Verification items for the finished model (mm, model axes). A direction names the side the tool comes from. Coordinates: 2 decimals unless noted, no trailing zeros. Order: outer loops, then holes, each group sorted by start corner. A loop starts at its lowest first (then second) coordinate and runs counter-clockwise, first axis right, second up. Notation, with made-up numbers: M 51,-29 L 108,-29 A24 cw 108,0 Z; hole C 25.5,-26 d10. An arc over 180 degrees is marked long. Return JSON: item names as keys, results as strings. Group by question number.
Q1. Section check D-D, the plane z = 19. Enter the section's corners in (x, y).
Q2. Access from +Z, -Z, +X, -X, +Y, -Y to the whole of each face (thin tool, end or side, straight path). Record for faces 4 (the face through (1.5, -0.9, 28.7)), 5 (the face through (-3.05, -0.04, 3.94)), 6 (the face through (2.37, -1.396, 29.72)), 7 (the face through (3, 1, 10)).
Q3. Mould release check, pull along X, two halves, no side actions. Record for faces 1 (the face through (-2.393, -1.354, 29.72)), 2 (the face through (-1.5, 0.9, 28.7)), 3 (the face through (0, -3, 0)): pulls with the +X half, pulls with the -X half, needs draft (parallel to the pull), parting line crosses it, or undercut.
Q4. Section check C-C, the plane y = 0.5. Enter the section's corners in (x, z), then the cut area to 3 significant figures.
Q5. Go/stop test with flat-tipped pins: pin 1 Ø1 at (y, z) = (1, 23) entering from -X; pin 2 Ø2 at (x, y) = (1, -1) entering from +Z; pin 3 Ø1.5 at (y, z) = (-1, 22.5) entering from -X; pin 4 Ø2 at (x, z) = (2, 35) entering from +Y. Record where each tip stops, or that it passes through.
Q6. Section check B-B, the plane x = 0. Enter the section's corners in (y, z), then the cut area to 3 significant figures.
Q7. Section check A-A, the plane z = 3.5. Enter the section's corners in (x, y).
Q8. Thickness scan on probe 1 along Y at (x, z) = (-0.25, 13); probe 2 along Y at (x, z) = (-1.5, 3); probe 3 along X at (y, z) = (0, 30). Record the ranges inside material, lowest first.
from build123d import *

# Parameters (mm, degrees)
BOSS_EXTRUDE2_DEPTH     = 10
CUT_EXTRUDE2_DEPTH      = 8
BOSS_EXTRUDE3_DEPTH     = 40
CUT_EXTRUDE3_DEPTH      = 51.268926784
CUT_EXTRUDE3_DEPTH_BACK = 51.268926784


with BuildPart() as part:
    # Sketch1 → Boss-Extrude2 (new body)
    with BuildSketch(Plane.XY):
        with BuildLine():
            Line((-2.416609195, 3.25), (2.416609195, 3.25))
            ThreePointArc((2.416609195, 3.25), (4.05, 0), (2.416609195, -3.25))
            Line((2.416609195, -3.25), (-2.416609195, -3.25))
            ThreePointArc((-2.416609195, -3.25), (-4.05, 0), (-2.416609195, 3.25))
        make_face()
    extrude(amount=BOSS_EXTRUDE2_DEPTH)

    # Sketch3 → Cut-Extrude2 (cut)
    with BuildSketch(Plane(origin=(0, 0, 0), x_dir=(-1, 0, 0), z_dir=(0, 0, -1))):
        with BuildLine():
            Line((2.059126028, 2.25), (-2.059126028, 2.25))
            ThreePointArc((-2.059126028, 2.25), (-3.05, 0), (-2.059126028, -2.25))
            Line((-2.059126028, -2.25), (2.059126028, -2.25))
            ThreePointArc((2.059126028, -2.25), (3.05, 0), (2.059126028, 2.25))
        make_face()
    extrude(amount=-CUT_EXTRUDE2_DEPTH, mode=Mode.SUBTRACT)

    # Sketch4 → Boss-Extrude3 (add)
    with BuildSketch(Plane.XY.offset(10)):
        Polygon((1.586062627, -2.750952322), (3.175425909, -0.001905634), (1.589363281, 2.749046688), (-1.586062627, 2.750952322), (-3.175425909, 0.001905634), (-1.589363281, -2.749046688), align=None)
    extrude(amount=BOSS_EXTRUDE3_DEPTH)

    # Sketch5 → Cut-Extrude3 (cut, two sides: drawn at the far end of the back side and taken through both)
    with BuildSketch(Plane.XY.offset(50).offset(-CUT_EXTRUDE3_DEPTH_BACK)):
        Polygon((-1.011412997, -1.749393347), (1.009312581, -1.750606023), (2.020725578, -0.001212676), (1.011412997, 1.749393347), (-1.009312581, 1.750606023), (-2.020725578, 0.001212676), align=None)
    extrude(amount=CUT_EXTRUDE3_DEPTH + CUT_EXTRUDE3_DEPTH_BACK, mode=Mode.SUBTRACT)


solid = part.part
Numbers:
{
 "1": {"outline": "M -3.18,0 L -1.59,-2.75 L 1.59,-2.75 L 3.18,0 L 1.59,2.75 L -1.59,2.75 Z; hole M -2.02,0 L -1.01,-1.75 L 1.01,-1.75 L 2.02,0 L 1.01,1.75 L -1.01,1.75 Z"},
 "2": {"face 4": "+Z, -Z", "face 5": "-Z", "face 6": "+Z, +X, -Y", "face 7": "+Z"},
 "3": {"face 1": "pulls with the -X half", "face 2": "undercut", "face 3": "needs draft"},
 "4": {"outline": "M -4.02,0 L -3.01,0 L -3.01,8 L -1.73,8 L -1.73,50 L -2.89,50 L -2.89,10 L -4.02,10 Z; M 1.73,8 L 3.01,8 L 3.01,0 L 4.02,0 L 4.02,10 L 2.89,10 L 2.89,50 L 1.73,50 Z", "area": "118 mm2"},
 "5": {"pin 1": "stops at x = -2.89", "pin 2": "stops at z = 50", "pin 3": "stops at x = -3.03", "pin 4": "stops at y = 2.75"},
 "6": {"outline": "M -3.25,0 L -2.25,0 L -2.25,8 L -1.75,8 L -1.75,50 L -2.75,50 L -2.75,10 L -3.25,10 Z; M 1.75,8 L 2.25,8 L 2.25,0 L 3.25,0 L 3.25,10 L 2.75,10 L 2.75,50 L 1.75,50 Z", "area": "102 mm2"},
 "7": {"outline": "M -2.42,-3.25 L 2.42,-3.25 A4.05 ccw 2.42,3.25 L -2.42,3.25 A4.05 ccw Z; hole M -2.06,-2.25 L 2.06,-2.25 A3.05 ccw 2.06,2.25 L -2.06,2.25 A3.05 ccw Z"},
 "8": {"probe 1": "y = -2.75 to -1.75, 1.75 to 2.75", "probe 2": "y = -3.25 to -2.25, 2.25 to 3.25", "probe 3": "x = -3.17 to -2.02, 2.02 to 3.17"}
}
